```python
from build123d import *

# Parameters (mm, degrees)
F2_R     = 4
F3_DEPTH = 25.4
F4_R     = 6.75
F4_R_2   = 4
F5_DEPTH = 8


with BuildPart() as f1:
    # F0 (on Front) → F1 (revolve)
    with BuildSketch(Plane.XZ):
        Polygon((-47.183853, 15.875), (10.1137, 15.875), (130.7637, 15.875), (135.7675, 15.875), (135.7675, 47.498), (130.7637, 47.498), (130.7637, 63.5), (111.7137, 63.5), (111.7137, 41.275), (10.1137, 41.275), (10.1137, 31.75), (-27.9863, 31.75), (-27.9863, 25.4), (-66.0863, 25.4), (-66.0863, 15.875), align=None)
    revolve(axis=Axis((0.887014, 0, 0), (1, 0, 0)))

    # F2 (on face) → F3 (cut)
    with BuildSketch(Plane.YZ.offset(130.7637)):
        with Locations((0, 54.0004)):
            Circle(F2_R)
        with Locations((46.765718, -27.0002)):
            Circle(F2_R)
        with Locations((-46.765718, -27.0002)):
            Circle(F2_R)
    extrude(amount=-F3_DEPTH, mode=Mode.SUBTRACT)

    # F4 (on face) → F5 (cut)
    with BuildSketch(Plane(origin=(111.7137, 0, 0), x_dir=(0, -1, 0), z_dir=(-1, 0, 0))):
        with Locations((0, 54.0004)):
            Circle(F4_R)
        with Locations((0, 54.0004)):
            Circle(F4_R_2, mode=Mode.SUBTRACT)
        with Locations((46.765718, -27.0002)):
            Circle(F4_R)
        with Locations((46.765718, -27.0002)):
            Circle(F4_R_2, mode=Mode.SUBTRACT)
        with Locations((-46.765718, -27.0002)):
            Circle(F4_R)
        with Locations((-46.765718, -27.0002)):
            Circle(F4_R_2, mode=Mode.SUBTRACT)
    extrude(amount=-F5_DEPTH, mode=Mode.SUBTRACT)


solid = f1.part
```
Verification items for the finished model (mm, model axes). A direction names the side the tool comes from. Coordinates: 2 decimals unless noted, no trailing zeros. Loops run counter-clockwise (first coordinate to the right, second up) from the corner with the lowest first, then second, coordinate; pieces in that order, holes last. Notation, with made-up numbers: (43, 48.5) -> (63, 48.5) arc R22 ccw to (63, 60.5) -> close; hole circle Ø6 at (35.5, 80.5). An arc over 180 degrees is marked (long way). Answer in a Markdown table with one row per item. Add a question column.
1. Material ranges on probe 1 along Z at (x, y) = (116.75, 0) (3 decimals); probe 2 along Y at (x, z) = (92, 0) (3 decimals); probe 3 along Y at (x, z) = (-33, 0.5), recorded low to high. Write a range as [from, to].
2. Access from +Z, -Z, +X, -X, +Y, -Y to the whole of each face (thin tool, end or side, straight path). Record for faces 4 (the face through (133.231, -14.267, 45.305)), 5 (the face through (125.32, 50.58, -25.8)), 6 (the face through (119.714, 46.9, -31.4)).
3. Section check C-C, the plane x = -32. Enter the section's corners in (y, z) (3 decimals), then the cut area to 3 significant figures.
4. Section check D-D, the plane z = 34. Enter the section's corners in (x, y).
5. Depth check by flat-ended pin: P1, Ø7, axis at y = 46.77, z = -27, coming from the -X side; P2, Ø4, axis at y = -1.5, z = -31, coming from the -X side; P3, Ø10, axis at x = 51.5, y = 15.5, coming from the -Z side; P4, Ø2, axis at y = -27.5, z = 21, coming from the -X side. Enter the tip coordinate at first touch or a pass-through.
6. Draft check along Y on faces 1 (the face through (111.714, -0.89, 41.44)), 2 (the face through (115.66, -3.63, 59.69)), 3 (the face through (60.202, 40.293, -8.948)). Enter one of: +Y half, -Y half, draft (parallel to the pull), parting line (faces both ways), or undercut.
7. Section check B-B, the plane x = -1. Enter the section's corners in (y, z) (3 decimals).
Derived:
| question | item | result |
|---|---|---|
| 1 | probe 1 | z = [-63.5, -15.875], [15.875, 47.25], [60.75, 63.5] |
| 1 | probe 2 | y = [-41.275, -15.875], [15.875, 41.275] |
| 1 | probe 3 | y = [-25.4, -15.87], [15.87, 25.4] |
| 2 | face 4 | +X |
| 2 | face 5 | +X, -X |
| 2 | face 6 | -X |
| 3 | outline | circle Ø50.8 at (0, 0); hole circle Ø31.75 at (0, 0) |
| 3 | area | 1,240 mm² |
| 4 | outline | (10.11, -23.4) -> (111.71, -23.4) -> (111.71, -53.63) -> (130.76, -53.63) -> (130.76, -33.17) -> (135.77, -33.17) -> (135.77, 33.17) -> (130.76, 33.17) -> (130.76, 53.63) -> (111.71, 53.63) -> (111.71, 23.4) -> (10.11, 23.4) -> close |
| 5 | P1 | passes through |
| 5 | P2 | stops at x = -27.99 |
| 5 | P3 | stops at z = -39.92 |
| 5 | P4 | stops at x = 10.11 |
| 6 | face 1 | draft |
| 6 | face 2 | undercut |
| 6 | face 3 | parting line |
| 7 | outline | circle Ø63.5 at (0, 0); hole circle Ø31.75 at (0, 0) |
